Could you check a few things on this drawing? It's one solid part, dimensions in mm from its lowest x, y, z. A direction names the side the tool comes from. Coordinates: 2 decimals unless noted, no trailing zeros. Loops run counter-clockwise (first coordinate to the right, second up) from the corner with the lowest first, then second, coordinate; pieces in that order, holes last. Notation, with made-up numbers: M 89,58.25 L 115,58.25 A22 ccw 115,81.25 Z; hole C 4,54 d2. An arc over 180 degrees is marked long. Answer as a JSON object with one key per item and string values. Group by question number.
Item 1: Suppose I cut it at D-D (y = 8). Write out the boundary of the cut face in (x, z).
Item 2: Which directions (+Z, -Z, +X, -X, +Y, -Y) give clear straight access to the entire face, cutting with the end or side of a thin tool? Please do the marked faces 1 and 2.
Item 3: Suppose I cut it at C-C (z = 33.5). Write out the boundary of the cut face in (x, y), then the cut area to 3 significant figures.
Item 4: Suppose I cut it at A-A (y = 50). Write out the boundary of the cut face in (x, z), then the cut area to 3 significant figures.
Item 5: If I drill on line 1 (Z direction, x = 86.5, y = 95); line 2 (X direction, y = 50, z = 36); line 3 (Y direction, x = 53, z = 24), over which ranges is the centre line in solid material (lowest first)?
Item 6: I'm going to push flat-ended pins straight in: pin 1 Ø2 at (y, z) = (45.5, 9) entering from -X; pin 2 Ø8 at (y, z) = (31, 24) entering from +X; pin 3 Ø1 at (x, z) = (47, 44) entering from -Y. Where does each tip first touch, or does it pass through?
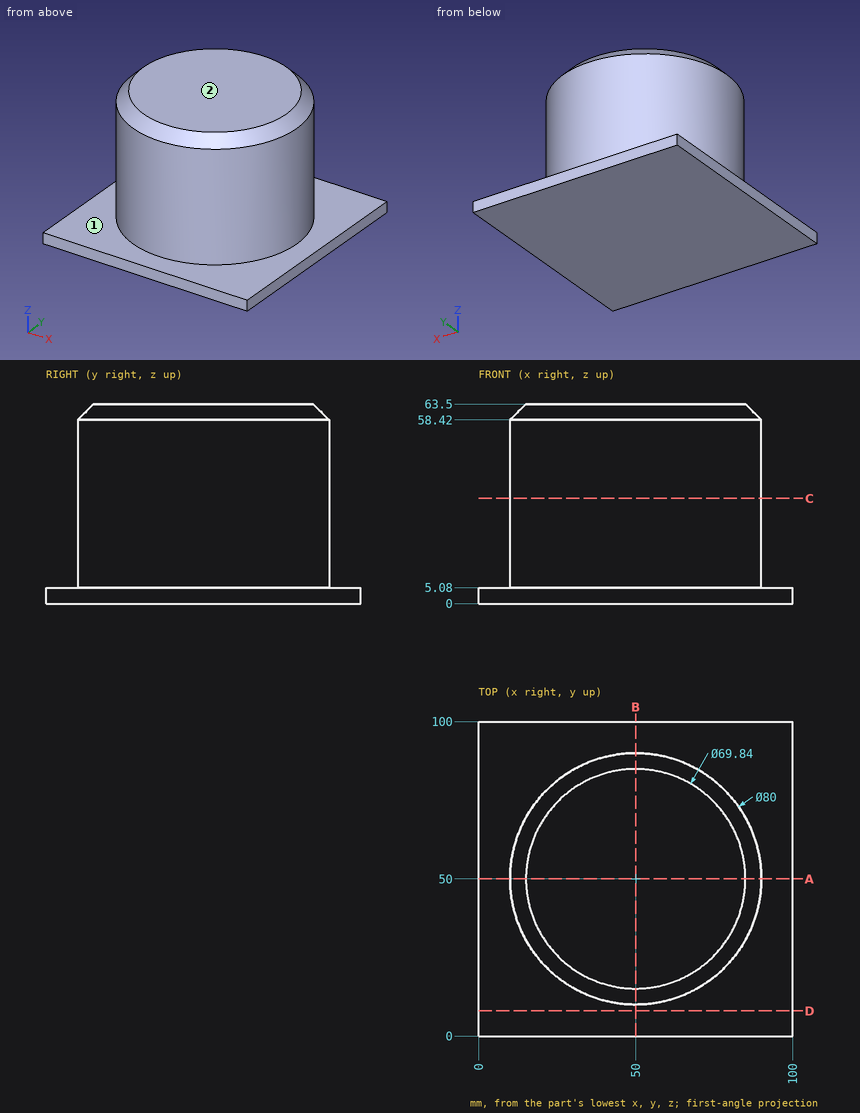
From the geometry:
{
 "1": {"outline": "M 0,0 L 100,0 L 100,5.08 L 0,5.08 Z"},
 "2": {"face 1": "+Z", "face 2": "+Z, +X, -X, +Y, -Y"},
 "3": {"outline": "C 50,50 d80", "area": "5,030 mm2"},
 "4": {"outline": "M 0,0 L 100,0 L 100,5.08 L 90,5.08 L 90,58.42 L 84.92,63.5 L 15.08,63.5 L 10,58.42 L 10,5.08 L 0,5.08 Z", "area": "5,160 mm2"},
 "5": {"line 1": "0 to 5.08", "line 2": "10 to 90", "line 3": "10.11 to 89.89"},
 "6": {"pin 1": "x = 10.15", "pin 2": "x = 87.08", "pin 3": "y = 10.08"}
}
